```python
from build123d import *

# Parameters (mm, degrees)
SKETCH2_OUTSIDE_W   = 34.314
SKETCH2_OUTSIDE_H   = 34.314
SKETCH2_OUTSIDE_W_2 = 16
SKETCH2_OUTSIDE_H_2 = 32.405240589
CUT_EXTRUDE1_DEPTH  = 20
SKETCH3_R           = 6
CUT_EXTRUDE2_DEPTH  = 40


with BuildPart() as part:
    # Sketch1 → Revolve1 (revolve)
    with BuildSketch(Plane.XY):
        with BuildLine():
            Line((0, 12), (0, -12))
            ThreePointArc((0, -12), (-12, 0), (0, 12))
        make_face()
    revolve(axis=Axis((0, 16.812644527, 0), (0, -1, 0)))

    # Sketch2 outside → Cut-Extrude1 (cut, symmetric)
    with BuildSketch(Plane.XY):
        Rectangle(SKETCH2_OUTSIDE_W, SKETCH2_OUTSIDE_H)
        with Locations((0, -1.599752384)):
            Rectangle(SKETCH2_OUTSIDE_W_2, SKETCH2_OUTSIDE_H_2, mode=Mode.SUBTRACT)
    extrude(amount=CUT_EXTRUDE1_DEPTH, both=True, mode=Mode.SUBTRACT)

    # Sketch3 → Cut-Extrude2 (cut)
    with BuildSketch(Plane.ZY.offset(8)):
        with Locations(Location((0, 0, 0), (0, 0, 270))):
            Circle(SKETCH3_R)
    extrude(amount=-CUT_EXTRUDE2_DEPTH, mode=Mode.SUBTRACT)


solid = part.part
```
Work out the finished part from the listing and answer in its coordinate system (mm). Give positions to 0.01 mm unless a question says otherwise; leave off trailing zeros. Order: outer loops, then holes, each group sorted by start corner. A loop starts at its lowest first (then second) coordinate and runs counter-clockwise, first axis right, second up. Notation, with made-up numbers: (13.5, 73) - (66.5, 73) arc R24 ccw to (66.5, 104) - close; hole circle Ø1 at (-6, -35). An arc over 180 degrees is marked (long way). One line per item, written item: value. Start each with the question number.
1. For a pull along Y with two mould halves and no side action, classify faces 1 (the face through (-0.112, -5.723, 1.802)), 2 (the face through (8, 2, -6)) as released by +Y, released by -Y, zero draft, split by the parting line, or undercut.
2. Each of these flat-tipped pins is pushed along its axis until it touches: pin 1 Ø8 at (x, y) = (-6, -0.5) entering from +Z; pin 2 Ø8 at (x, z) = (1.5, 4.5) entering from -Y; pin 3 Ø1 at (x, z) = (0.5, 8) entering from +Y (3 decimals); pin 4 Ø9.5 at (y, z) = (0, 0) entering from +X. Where does it stop, or does it pass through?
3. Consider line 1 (Z direction, x = 0, y = 0); line 2 (Z direction, x = 4.75, y = 0.5); line 3 (Y direction, x = 2.5, z = -2.25). Determine where each line is inside the solid, lowest interval first.
4. Section C-C, the plane x = -2.75 is taken. Write down the section's boundary in (y, z).
5. Section D-D, the plane z = 9.5 is taken. Write down the section's boundary in (x, y).
6. Section A-A, the plane z = 0 is taken. Write down the section's boundary in (x, y).
Filled sheet:
1. face 1: undercut
1. face 2: zero draft
2. pin 1: z = 11.83
2. pin 2: y = -11.98
2. pin 3: y = 9.355
2. pin 4: through
3. line 1: -12 to -6, 6 to 12
3. line 2: -11.01 to -5.98, 5.98 to 11.01
3. line 3: -11.52 to -5.56, 5.56 to 11.52
4. outline: circle Ø23.36 at (0, 0); hole circle Ø12 at (0, 0)
5. outline: circle Ø14.66 at (0, 0)
6. outline: (-8, -8.94) arc R12 ccw to (8, -8.94) - (8, -6) - (-8, -6) - close; (-8, 6) - (8, 6) - (8, 8.94) arc R12 ccw to (-8, 8.94) - close
